Read the model definition and answer for the solid it produces. Units are mm, in the model's axes. Give positions to 0.01 mm unless a question says otherwise; leave off trailing zeros. Order: outer loops, then holes, each group sorted by start corner. A loop starts at its lowest first (then second) coordinate and runs counter-clockwise, first axis right, second up. Notation, with made-up numbers: (64.25, 5.5) - (91.25, 5.5) arc R13 cw to (91.25, 12.5) - close; hole circle Ø6 at (68, 20.25). An arc over 180 degrees is marked (long way). Use a Markdown table: item, result. Add a question column.
1. Consider L1, parallel to Y at x = -2.5, z = 0.65; L2, parallel to Y at x = -5.25, z = 0.5; L3, parallel to X at y = 9, z = 1.4. Determine where each line is inside the solid, lowest interval first.
2. A cutting plane is placed at B-B on z = 0.45. State how many separate pieces and enclosed holes the cut face has, and give its area (3 significant figures).
3. Flat-ended cylindrical pins translate along their axes: P1, Ø0.8, axis at y = 12, z = 1, coming from the -X side; P2, Ø1, axis at x = -1.5, y = -29.5, coming from the -Z side. Find the tip coordinate at first contact, or state that the pin passes through.
4. A cutting plane is placed at A-A on x = -2.5. Determine the outline of the cut face in (y, z), and give its area (4 significant figures).
```python
from build123d import *

# Parameters (mm, degrees)
F1_DEPTH    = 1.5
F2_T1_DEPTH = 6.5
F2_T3_DEPTH = 6.4616050658
F3_R        = 2
F4_R        = 3


# Not quite as in the source:
# - a fillet or chamfer that OpenCascade refuses, or shapes differently, is made with other operations: its cross-section is extruded or revolved along the edge and cut away or added


with BuildPart() as f1:
    # F0 (on Top) → F1 (new body)
    with BuildSketch(Plane.XY):
        with BuildLine():
            Line((6.7359172925, 27.2759429877), (-4.7640827075, 27.2759429877))
            ThreePointArc((-4.7640827075, 27.2759429877), (-5.4711894887, 26.9830497689), (-5.7640827075, 26.2759429877))
            Line((-5.7640827075, 26.2759429877), (-5.7640827075, 18.2759429877))
            ThreePointArc((-5.7640827075, 18.2759429877), (-5.4711894887, 17.5688362065), (-4.7640827075, 17.2759429877))
            Line((-4.7640827075, 17.2759429877), (-3.7640827075, 17.2759429877))
            Line((-3.7640827075, 17.2759429877), (-3.7640827075, 19.2759429877))
            Line((-3.7640827075, 19.2759429877), (7.2359172925, 19.2759429877))
            Line((7.2359172925, 19.2759429877), (7.2359172925, 17.2759429877))
            Line((7.2359172925, 17.2759429877), (7.2359172925, 16.2759429877))
            Line((7.2359172925, 16.2759429877), (7.2359172925, 14.2759429877))
            Line((7.2359172925, 14.2759429877), (-3.8877718616, 14.2759429877))
            Line((-3.8877718616, 14.2759429877), (-3.8877718616, 16.2759429877))
            Line((-3.8877718616, 16.2759429877), (-4.7640827075, 16.2759429877))
            ThreePointArc((-4.7640827075, 16.2759429877), (-5.4711894887, 15.9830497689), (-5.7640827075, 15.2759429877))
            Line((-5.7640827075, 15.2759429877), (-5.7640827075, 7.2759429877))
            ThreePointArc((-5.7640827075, 7.2759429877), (-5.4711894887, 6.5688362065), (-4.7640827075, 6.2759429877))
            Line((-4.7640827075, 6.2759429877), (6.7359172925, 6.2759429877))
            ThreePointArc((6.7359172925, 6.2759429877), (7.0894706831, 6.1294963783), (7.2359172925, 5.7759429877))
            ThreePointArc((7.2359172925, 5.7759429877), (7.0894706831, 5.4223895971), (6.7359172925, 5.2759429877))
            Line((6.7359172925, 5.2759429877), (-5.7640827075, 5.2759429877))
            Line((-5.7640827075, 5.2759429877), (-6.7640827075, 5.2759429877))
            Line((-6.7640827075, 5.2759429877), (-6.7640827075, -47.2240570123))
            Line((-6.7640827075, -47.2240570123), (9.2359172925, -47.2240570123))
            Line((9.2359172925, -47.2240570123), (9.2359172925, 80.7759429877))
            Line((9.2359172925, 80.7759429877), (-6.7640827075, 80.7759429877))
            Line((-6.7640827075, 80.7759429877), (-6.7640827075, 28.2759429877))
            Line((-6.7640827075, 28.2759429877), (-5.7640827075, 28.2759429877))
            Line((-5.7640827075, 28.2759429877), (6.7359172925, 28.2759429877))
            ThreePointArc((6.7359172925, 28.2759429877), (7.0894706831, 28.1294963783), (7.2359172925, 27.7759429877))
            ThreePointArc((7.2359172925, 27.7759429877), (7.0894706831, 27.4223895971), (6.7359172925, 27.2759429877))
        make_face()
        with BuildLine():
            ThreePointArc((-4.7640827075, -44.2240570123), (-4.4711894887, -43.5169502311), (-3.7640827075, -43.2240570123))
            Line((-3.7640827075, -43.2240570123), (6.2359172925, -43.2240570123))
            ThreePointArc((6.2359172925, -43.2240570123), (6.9430240737, -43.5169502311), (7.2359172925, -44.2240570123))
            ThreePointArc((7.2359172925, -44.2240570123), (6.9430240737, -44.9311637935), (6.2359172925, -45.2240570123))
            Line((6.2359172925, -45.2240570123), (-3.7640827075, -45.2240570123))
            ThreePointArc((-3.7640827075, -45.2240570123), (-4.4711894887, -44.9311637935), (-4.7640827075, -44.2240570123))
        make_face(mode=Mode.SUBTRACT)
        with BuildLine():
            Line((6.2359172925, 76.7759429877), (-3.7640827075, 76.7759429877))
            ThreePointArc((-3.7640827075, 76.7759429877), (-4.4711894887, 77.0688362065), (-4.7640827075, 77.7759429877))
            ThreePointArc((-4.7640827075, 77.7759429877), (-4.4711894887, 78.4830497689), (-3.7640827075, 78.7759429877))
            Line((-3.7640827075, 78.7759429877), (6.2359172925, 78.7759429877))
            ThreePointArc((6.2359172925, 78.7759429877), (6.9430240737, 78.4830497689), (7.2359172925, 77.7759429877))
            ThreePointArc((7.2359172925, 77.7759429877), (6.9430240737, 77.0688362065), (6.2359172925, 76.7759429877))
        make_face(mode=Mode.SUBTRACT)
    extrude(amount=F1_DEPTH)

    # F2: fillet of radius 1 on 2 edges, made by hand

    # F2_s2 → F2_t1 (cut)
    with BuildSketch(Plane.XY.offset(-2.5)):
        with BuildLine():
            ThreePointArc((-3.7640827075, 18.2759429877), (-4.0569759263, 17.5688362065), (-4.7640827075, 17.2759429877))
            Line((-4.7640827075, 17.2759429877), (-3.7640827075, 17.2759429877))
            Line((-3.7640827075, 17.2759429877), (-3.7640827075, 18.2759429877))
        make_face()
    extrude(amount=F2_T1_DEPTH, mode=Mode.SUBTRACT)

    # F2_s4 → F2_t3 (cut)
    with BuildSketch(Plane.XY.offset(-2.4808025329)):
        with BuildLine():
            ThreePointArc((-4.7640827075, 16.2759429877), (-4.1382089376, 15.94555507), (-3.8877718616, 15.2836219745))
            Line((-3.8877718616, 15.2836219745), (-3.8877718616, 16.2759429877))
            Line((-3.8877718616, 16.2759429877), (-4.7640827075, 16.2759429877))
        make_face()
    extrude(amount=F2_T3_DEPTH, mode=Mode.SUBTRACT)

    # F3
    f3_edges = [f1.edges().sort_by_distance(p)[0] for p in [
        (-6.764083, 28.275943, 0.75),
        (-6.764083, 5.275943, 0.75),
    ]]
    fillet(f3_edges, radius=F3_R)

    # F4
    f4_edges = [f1.edges().sort_by_distance(p)[0] for p in [
        (9.235917, 80.775943, 0.75),
        (-6.764083, 80.775943, 0.75),
        (-6.764083, -47.224057, 0.75),
        (9.235917, -47.224057, 0.75),
    ]]
    fillet(f4_edges, radius=F4_R)


solid = f1.part
```
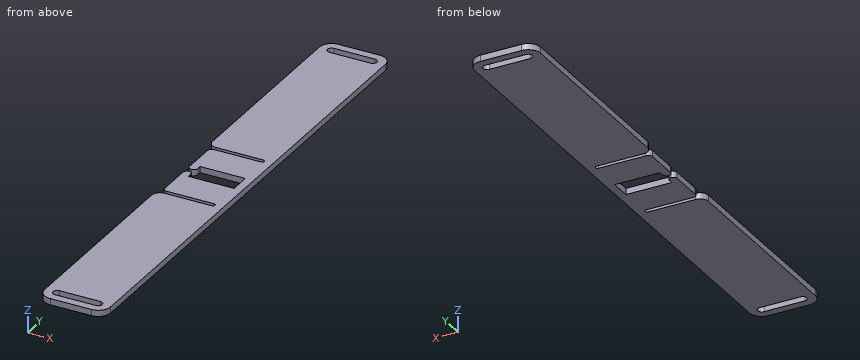
Output values:
| question | item | result |
|---|---|---|
| 1 | L1 | -47.22 to -45.22, -43.22 to 5.28, 6.28 to 14.28, 19.28 to 27.28, 28.28 to 76.78, 78.78 to 80.78 |
| 1 | L2 | -46.83 to 5.22, 6.4 to 16.15, 17.4 to 27.15, 28.34 to 80.38 |
| 1 | L3 | -5.76 to 9.24 |
| 2 | separate pieces | 1 |
| 2 | enclosed holes | 2 |
| 2 | area | 1,880 mm² |
| 3 | P1 | x = -5.76 |
| 3 | P2 | z = 0 |
| 4 | outline | (-47.22, 0) - (-45.22, 0) - (-45.22, 1.5) - (-47.22, 1.5) - close; (-43.22, 0) - (5.28, 0) - (5.28, 1.5) - (-43.22, 1.5) - close; (6.28, 0) - (14.28, 0) - (14.28, 1.5) - (6.28, 1.5) - close; (19.28, 0) - (27.28, 0) - (27.28, 1.5) - (19.28, 1.5) - close; (28.28, 0) - (76.78, 0) - (76.78, 1.5) - (28.28, 1.5) - close; (78.78, 0) - (80.78, 0) - (80.78, 1.5) - (78.78, 1.5) - close |
| 4 | area | 175.5 mm² |
